Source: CAD feature listing. Evaluate the final solid. Frame: model axes, mm. A direction names the side the tool comes from. Round coordinates to 2 decimals unless told otherwise and drop trailing zeros. Loops run counter-clockwise (first coordinate to the right, second up) from the corner with the lowest first, then second, coordinate; pieces in that order, holes last.
Item 1: Ray query, L1, parallel to Z at x = 0, y = 1.45; L2, parallel to Z at x = 77.5, y = 24; L3, parallel to X at y = 7.5, z = 62.5. Return the intervals inside material, ascending.
Item 2: Section query C-C on y = 30. Return loops of the section in (x, z), then the cut area to 3 significant figures.
Item 3: Section query B-B on x = -62. Return loops of the section in (y, z), then the cut area to 3 significant figures.
Item 4: Pull-direction query (Z, two-part tool) for faces 1 (the flat face through (1, 0, 1)), 2 (the cylindrical face through (84.005, 21.759, -40.924)), 3 (the cylindrical face through (-20.244, 1.521, 46.192)); classes: released by +Z, released by -Z, zero draft, split by the parting line, or undercut.
Item 5: First-contact query: P1, Ø1, axis at y = 10.5, z = -9.5, coming from the -X side; P2, Ø3.5, axis at x = -29.7, z = -8.49, coming from the +Y side; P3, Ø10, axis at x = -38.5, y = 24, coming from the +Z side. Flat tips, straight axial feed; report the tip coordinate or a pass-through.
Item 6: Section query A-A on z = 45. Return loops of the section in (x, y), then the cut area to 3 significant figures.
Item 7: Access query for faces 4 (the cylindrical face through (-14.87, 21.76, -88.72)), 5 (the flat face through (-63.049, 1.521, 57.498)). Directions: +Z, -Z, +X, -X, +Y, -Y. A direction counts if a zero-diameter tool reaches every point of the face in a straight line with its end or side. Return the directions, or none.
Autodesk Inventor part; units mm, degrees
ref_plane "YZ Plane" through (0, 0, 0) normal (1, 0, 0) x (0, 1, 0)
ref_plane "XZ Plane" through (0, 0, 0) normal (0, 1, 0) x (-1, 0, 0)
ref_plane "XY Plane" through (0, 0, 0) normal (0, 0, 1) x (1, 0, 0)
sketch "Sketch1" plane through (0, 0, 0) normal (0, 1, 0) x (-1, 0, 0)
  circle A0 centre (0, 0) radius 100
  dimension "d0" = 200
extrude "Extrusion1" add sketch "Sketch1" along normal blind 40
sketch "Sketch3" plane through (0, 40, 0) normal (0, 1, 0) x (1, 0, 0)
  circle A0 centre (0, 0) radius 97
  circle A1 centre (0, 0) radius 100
  dimension "d14" = 3
extrude "Extrusion3" cut sketch "Sketch3" against normal blind 37 contours A0
sketch "Sketch6" plane through (0, 40, 0) normal (0, 1, 0) x (1, 0, 0)
  circle A0 centre (65.0538, -65.0538) radius 2.2
  line L0 (0, 0) -> (65.0538, -65.0538)
  line L1 (0, 0) -> (0, 29.3697)
  arc A1 (68.5894, -61.5183) -> (61.5183, -68.5894) centre (65.0538, -65.0538) ccw
  line L2 (61.5183, -68.5894) -> (64.9626, -72.0337)
  line L3 (68.5894, -61.5183) -> (72.0337, -64.9626)
  arc A2 (79.7026, 46.2222) -> (84.2426, 37.3121) centre (81.9726, 41.7671) ccw
  circle A3 centre (81.9726, 41.7671) radius 2.2
  line L4 (84.2426, 37.3121) -> (88.5827, 39.5235)
  line L5 (79.7026, 46.2222) -> (84.0428, 48.4336)
  arc A4 (-19.3304, 90.0852) -> (-9.4535, 91.6495) centre (-14.392, 90.8673) ccw
  circle A5 centre (-14.392, 90.8673) radius 2.2
  line L6 (-9.4535, 91.6495) -> (-10.2155, 96.4606)
  line L7 (-19.3304, 90.0852) -> (-20.0924, 94.8962)
  arc A6 (-91.6495, 9.4535) -> (-90.0852, 19.3304) centre (-90.8673, 14.392) ccw
  circle A7 centre (-90.8673, 14.392) radius 2.2
  line L8 (-90.0852, 19.3304) -> (-94.8962, 20.0924)
  line L9 (-91.6495, 9.4535) -> (-96.4606, 10.2155)
  arc A8 (-37.3121, -84.2426) -> (-46.2222, -79.7026) centre (-41.7671, -81.9726) ccw
  circle A9 centre (-41.7671, -81.9726) radius 2.2
  line L10 (-46.2222, -79.7026) -> (-48.4336, -84.0428)
  line L11 (-37.3121, -84.2426) -> (-39.5235, -88.5827)
  circle A10 centre (0, 0) radius 97
  dimension "d106" = 4.4
  dimension "d109" = 92
  dimension "d111" = 135
  dimension "d112" = 10
  dimension "d115" = 360
extrude "Extrusion6" add sketch "Sketch6" against normal up to surface (37 mm away) contours A1 L3 A10 L2 | A10 L10 A8 L11 | L4 A2 L5 A10 | A10 L8 A6 L9 | L6 A4 L7 A10
sketch "Sketch9" plane through (0, 3, 0) normal (0, 1, 0) x (1, 0, 0)
  circle A0 centre (37.4767, 71.4178) radius 1.75
  circle A1 centre (7.7782, 41.7193) radius 1.75
  circle A2 centre (71.4178, 37.4767) radius 1.75
  circle A3 centre (41.7193, 7.7782) radius 1.75
  line L0 (0, 0) -> (0, 0)
  line L1 (0, 0) -> (-23.1827, 0)
  line L2 (0, 0) -> (0, 0)
  dimension "d115" = 360
  dimension "d77" = 42
  dimension "d78" = 48
  dimension "d79" = 42
  dimension "d80" = 48
  dimension "d81" = 135
  dimension "d82" = 24
  dimension "d83" = 24
  dimension "d84" = 24
  dimension "d85" = 3.5
  dimension "d86" = 3.5
  dimension "d87" = 3.5
  dimension "d88" = 3.5
  dimension "d89" = 35
extrude "Extrusion9" cut sketch "Sketch9" against normal blind 4
sketch "Sketch18" plane through (0, 3, 0) normal (0, 1, 0) x (1, 0, 0)
  line L0 (54.624, -13.2583) -> (13.2583, -54.624)
  line L1 (13.2583, -54.624) -> (31.643, -73.0088)
  line L2 (31.643, -73.0088) -> (73.0088, -31.643)
  line L3 (73.0088, -31.643) -> (54.624, -13.2583)
  line L4 (0, 0) -> (3.812, 0)
  line L5 (0, 0) -> (33.9411, -33.9411)
  circle A0 centre (54.624, -13.2583) radius 1.15
  circle A1 centre (73.0088, -31.643) radius 1.15
  circle A2 centre (13.2583, -54.624) radius 1.15
  circle A3 centre (31.643, -73.0088) radius 1.15
  line L6 (3.5355, -49.4975) -> (36.7696, -82.7315)
  line L7 (36.7696, -82.7315) -> (82.7315, -36.7696)
  line L8 (82.7315, -36.7696) -> (49.4975, -3.5355)
  line L9 (49.4975, -3.5355) -> (3.5355, -49.4975)
  dimension "d193" = 45
  dimension "d194" = 2.3
  dimension "d195" = 2.3
  dimension "d196" = 2.3
  dimension "d197" = 2.3
  dimension "d198" = 48
  dimension "d199" = 26
  dimension "d200" = 58.5
  dimension "d201" = 47
  dimension "d202" = 10.5
  dimension "d203" = 65
  dimension "d204" = 32.5
extrude "Extrusion11" cut sketch "Sketch18" against normal blind 10 contours L3 A0 L0 | L0 A0 L3 | A1 L2 L3 | L3 L2 A1 | A2 L1 L0 | L0 L1 A2 | A3 L1 L2 | L2 L1 A3
sketch "Sketch12" plane through (0, 3, 0) normal (0, 1, 0) x (1, 0, 0)
  circle A0 centre (-73.0088, 31.643) radius 1.15
  circle A1 centre (-54.624, 13.2583) radius 1.15
  circle A2 centre (-31.643, 73.0088) radius 1.15
  circle A3 centre (-13.2583, 54.624) radius 1.15
  line L0 (-54.624, 13.2583) -> (-73.0088, 31.643)
  line L1 (-73.0088, 31.643) -> (-31.643, 73.0088)
  line L2 (-31.643, 73.0088) -> (-13.2583, 54.624)
  line L3 (-13.2583, 54.624) -> (-54.624, 13.2583)
  line L4 (0, 0) -> (-33.9411, 33.9411)
  line L5 (0, 0) -> (28.9474, 0)
  line L6 (-3.5355, 49.4975) -> (-49.4975, 3.5355)
  line L7 (-49.4975, 3.5355) -> (-82.7315, 36.7696)
  line L8 (-82.7315, 36.7696) -> (-36.7696, 82.7315)
  line L9 (-36.7696, 82.7315) -> (-3.5355, 49.4975)
  dimension "d132" = 135
  dimension "d133" = 58.5
  dimension "d134" = 26
  dimension "d135" = 48
  dimension "d138" = 2.3
  dimension "d139" = 2.3
  dimension "d140" = 2.3
  dimension "d141" = 2.3
  dimension "d219" = 47
  dimension "d220" = 65
  dimension "d221" = 32.5
  dimension "d222" = 10.5
extrude "Extrusion12" cut sketch "Sketch12" against normal blind 10 contours A0 L0 L1 | L1 L0 A0 | L1 L2 A2 | A2 L2 L1 | L0 L3 A1 | A1 L3 L0 | L2 L3 A3 | A3 L3 L2
sketch "Sketch13" plane through (0, 3, 0) normal (0, 1, 0) x (1, 0, 0)
  circle A0 centre (-3.8891, -13.7886) radius 1.15
  circle A1 centre (13.7886, 3.8891) radius 1.15
  circle A2 centre (13.7886, -31.4663) radius 1.15
  circle A3 centre (31.4663, -13.7886) radius 1.15
  line L0 (13.7886, 3.8891) -> (31.4663, -13.7886)
  line L1 (13.7886, 3.8891) -> (-3.8891, -13.7886)
  line L2 (-3.8891, -13.7886) -> (13.7886, -31.4663)
  line L3 (13.7886, -31.4663) -> (31.4663, -13.7886)
  line L4 (0, 0) -> (4.9497, -4.9497)
  line L5 (0, 0) -> (0, 15.8788)
  circle A4 centre (-54.624, 13.2583) radius 1.15
  circle A5 centre (-13.2583, 54.624) radius 1.15
  line L6 (-54.624, 13.2583) -> (-13.2583, 54.624)
  dimension "d142" = 25
  dimension "d143" = 25
  dimension "d146" = 7
  dimension "d147" = 2.3
  dimension "d148" = 2.3
  dimension "d149" = 2.3
  dimension "d150" = 2.3
  dimension "d218" = 225
extrude "Extrusion13" cut sketch "Sketch13" against normal blind 10 contours A0 L2 L1 | L1 L2 A0 | L2 L3 A2 | A2 L3 L2 | L1 L0 A1 | A1 L0 L1 | L3 L0 A3 | A3 L0 L3
sketch "Sketch14" plane through (0, 3, 0) normal (0, 1, 0) x (1, 0, 0)
  circle A0 centre (-15.5563, -5.6569) radius 1.15
  circle A1 centre (-29.6985, 8.4853) radius 1.15
  circle A2 centre (5.6569, 15.5563) radius 1.15
  circle A3 centre (-8.4853, 29.6985) radius 1.15
  line L0 (-15.5563, -5.6569) -> (-29.6985, 8.4853)
  line L1 (-29.6985, 8.4853) -> (-8.4853, 29.6985)
  line L2 (-8.4853, 29.6985) -> (5.6569, 15.5563)
  line L3 (5.6569, 15.5563) -> (-15.5563, -5.6569)
  line L4 (0, 0) -> (-4.9497, 4.9497)
  line L5 (0, 0) -> (0, -29.7701)
  circle A4 centre (13.2583, -54.624) radius 1.15
  circle A5 centre (54.624, -13.2583) radius 1.15
  line L6 (13.2583, -54.624) -> (54.624, -13.2583)
  dimension "d153" = 20
  dimension "d154" = 30
  dimension "d155" = 2.3
  dimension "d156" = 2.3
  dimension "d157" = 2.3
  dimension "d158" = 2.3
  dimension "d160" = 7
  dimension "d217" = 225
extrude "Extrusion14" cut sketch "Sketch14" against normal blind 10 contours A0 L0 L3 | L3 L0 A0 | L0 L1 A1 | A1 L1 L0 | L3 L2 A2 | A2 L2 L3 | L1 L2 A3 | A3 L2 L1
sketch "Sketch16" plane through (0, 3, 0) normal (0, 1, 0) x (1, 0, 0)
  circle A0 centre (0, 80.5) radius 1.75
  circle A1 centre (0, 90.5) radius 1.75
  circle A2 centre (0, 0) radius 100
  line L0 (0, 100) -> (0, 80.5)
  dimension "d179" = 3.5
  dimension "d180" = 19.5
  dimension "d181" = 9.5
  dimension "d182" = 3.5
extrude "Extrusion16" cut sketch "Sketch16" against normal blind 10 contours A0 | A1 L0 | L0 A1
pattern_circular "Circular Pattern4" count 4 over 360 about axis through (0, -10, 0) along (0, 1, 0) of "Extrusion16"
sketch "Sketch17" plane through (0, 3, 0) normal (0, 1, 0) x (1, 0, 0)
  line L0 (0, 0) -> (-53.033, -53.033)
  line L1 (-53.033, -53.033) -> (-67.1751, -38.8909)
  line L2 (0, 0) -> (-22.9121, 0)
  line L3 (0, 0) -> (-42.4264, 42.4264)
  circle A0 centre (-42.4264, 42.4264) radius 22.5
  circle A1 centre (-42.4264, -42.4264) radius 22.5
  circle A2 centre (42.4264, -42.4264) radius 22.5
  circle A3 centre (42.4264, 42.4264) radius 22.5
  line L4 (-69.6063, -24.0892) -> (-46.0732, -20.2239)
  line L5 (-73.6535, -52.4198) -> (-52.144, -62.7197)
  arc A4 (-69.6063, -24.0892) -> (-73.6535, -52.4198) centre (-67.1751, -38.8909) ccw
  point P0 (-64.8915, -41.1745)
  point P1 (-26.5165, -26.5165)
  dimension "d188" = 45
  dimension "d189" = 75
  dimension "d190" = 20
  dimension "d207" = 60
  dimension "d208" = 45
  dimension "d209" = 45
  dimension "d212" = 360
  dimension "d216" = 15
extrude "Extrusion18" cut sketch "Sketch17" against normal blind 10
sketch "Sketch20" plane through (0, 3, 0) normal (0, 1, 0) x (1, 0, 0)
  line L0 (0, 0) -> (-22.6274, 22.6274)
  line L1 (-22.6274, 22.6274) -> (-29.7758, 15.479)
  line L2 (-22.6274, 22.6274) -> (-15.6337, 29.6211)
  line L3 (0, 0) -> (9.6667, 0)
  circle A0 centre (-29.7758, 15.479) radius 1.75
  circle A1 centre (-15.6337, 29.6211) radius 1.75
  circle A2 centre (-68.5894, 47.3762) radius 1.75
  circle A3 centre (-47.3762, 68.5894) radius 1.75
  line L4 (-68.5894, 47.3762) -> (-47.3762, 68.5894)
  line L5 (-57.9828, 57.9828) -> (-22.6274, 22.6274)
  dimension "d223" = 135
  dimension "d224" = 3.5
  dimension "d225" = 3.5
  dimension "d226" = 20
  dimension "d227" = 32
  dimension "d228" = 30
  dimension "d229" = 3.5
  dimension "d230" = 3.5
  dimension "d231" = 50
extrude "Extrusion19" cut sketch "Sketch20" against normal blind 10 contours A2 | A3
properties part number "RL_spider_center_mid_v3"
Data:
1. L1: z = -100 to -92.25, -88.75 to -82.25, -78.75 to 78.75, 82.25 to 88.75, 92.25 to 100
1. L2: z = -63.2 to -58.33, -44 to -39.53, 58.33 to 63.2
1. L3: x = -78.06 to -74.18, 60.76 to 69.57, 74.18 to 78.06
2. outline: circle Ø200 at (0, 0); hole (-96.46, -10.22) - (-91.65, -9.45) arc R5 cw to (-90.09, -19.33) - (-94.9, -20.09) arc R97 ccw to (-20.09, -94.9) - (-19.33, -90.09) arc R5 cw to (-9.45, -91.65) - (-10.22, -96.46) arc R97 ccw to (84.04, -48.43) - (79.7, -46.22) arc R5 cw to (84.24, -37.31) - (88.58, -39.52) arc R97 ccw to (72.03, 64.96) - (68.59, 61.52) arc R5 cw to (61.52, 68.59) - (64.96, 72.03) arc R97 ccw to (-39.52, 88.58) - (-37.31, 84.24) arc R5 cw to (-46.22, 79.7) - (-48.43, 84.04) arc R97 ccw to start; hole circle Ø4.4 at (-90.87, -14.39); hole circle Ø4.4 at (-41.77, 81.97); hole circle Ø4.4 at (-14.39, -90.87); hole circle Ø4.4 at (65.05, 65.05); hole circle Ø4.4 at (81.97, -41.77)
2. area: 2,220 mm2
3. outline: (0, -78.46) - (40, -78.46) - (40, -74.6) - (3, -74.6) - (3, -53.52) - (0, -53.52) - close; (0, -31.33) - (3, -31.33) - (3, 22.84) - (0, 22.84) - close; (0, 58) - (3, 58) - (3, 74.6) - (40, 74.6) - (40, 78.46) - (0, 78.46) - close
3. area: 584 mm2
4. face 1: zero draft
4. face 2: undercut
4. face 3: undercut
5. P1: stops at x = -99.59
5. P2: stops at y = 3
5. P3: stops at z = 94.22
6. outline: (-89.3, 0) - (-80.87, 0) - (-80.87, 3) - (-85.93, 3) - (-85.93, 40) - (-89.3, 40) - close; (-20.07, 0) - (20.07, 0) - (20.07, 3) - (-20.07, 3) - close; (64.78, 0) - (89.3, 0) - (89.3, 40) - (85.93, 40) - (85.93, 3) - (64.78, 3) - close
6. area: 469 mm2
7. face 4: +Y
7. face 5: +Y, -Y
